Read the model definition and answer for the solid it produces. Units are mm, in the model's axes. A direction names the side the tool comes from. Coordinates: 2 decimals unless noted, no trailing zeros. Write each loop counter-clockwise with the first axis right and the second up, starting at its lowest first coordinate (ties: lowest second). Pieces come first, ordered by that corner, then holes.
(1) The part is cut by section C-C, the plane x = -3.5. Determine the outline of the cut face in (y, z), and give its area (3 significant figures).
(2) Straight lines are drawn through the part: line 1 along X through (y, z) = (-6, 5.5); line 2 along Z through (x, y) = (3, -7.25); line 3 along X through (y, z) = (-10, -0.25). For each, find the intervals that lie inside material, in ascending order.
(3) Given pin 1 (0.6 mm diameter, centred on x = -6, z = -5.5, fed in from -Y); pin 2 (0.5 mm diameter, centred on x = -6, z = 1.5, fed in from -Y); pin 3 (3 mm diameter, centred on x = -10.5, z = 2.5, fed in from -Y), each flat-ended and moving along its own axis, determine where each tip first touches the part or whether it passes through.
(4) Which of the six approach directions +Z, -Z, +X, -X, +Y, -Y give full straight-line access (tool end or side, diameter ignored) to faces 1 (the flat face through (-21, -7, 0)), 2 (the flat face through (-19, -6, -5.3)), 3 (the flat face through (0, 0, 0))?
(5) The part is cut by section B-B, the plane y = -4. Determine the outline of the cut face in (x, z), and give its area (3 significant figures).
(6) The part is cut by section A-A, the plane y = -6. State how many separate pieces and enclosed holes the cut face has, and give its area (3 significant figures).
(7) Determine the mould class of faces 4 (the flat face through (6.3, -4, 0)), 5 (the flat face through (3.16, -13, 7.15)) for opening direction Z: pulls with the +Z half, pulls with the -Z half, needs draft (parallel to the pull), parting line crosses it, or undercut.
(8) The part is cut by section D-D, the plane z = -1. Determine the outline of the cut face in (x, y).
```python
from build123d import *

# Parameters (mm, degrees)
SKETCH_1_W                             = 44
SKETCH_1_H                             = 16
EXTRUDE_1_DEPTH                        = 2
SKETCH_2_W                             = 44
SKETCH_2_H                             = 16
SKETCH_2_W_2                           = 40
SKETCH_2_H_2                           = 12
EXTRUDE_2_DEPTH                        = 10
SKETCH_3_W                             = 5.5
SKETCH_3_H                             = 4
CUT_EXTRUDE_1_DEPTH                    = 2
SKETCH_4_W                             = 1.7
SKETCH_4_H                             = 12
EXTRUDE_4_DEPTH                        = 4.6
SKETCH_9_W                             = 44
SKETCH_9_H                             = 16
SKETCH_9_W_2                           = 42
SKETCH_9_H_2                           = 14
EXTRUDE_5_DEPTH                        = 1
SKETCH_12_W                            = 1
SKETCH_12_H                            = 12
CUT_EXTRUDE_3_DEPTH                    = 5
SKETCH_13_W                            = 41.2
SKETCH_13_H                            = 13.2
SKETCH_13_W_2                          = 40
SKETCH_13_H_2                          = 12
REVB_ASSEMBLYCLEARANCE_41P2X13P2_DEPTH = 11
SKETCH_14_W                            = 11
SKETCH_14_H                            = 7
REVB_USB_TOPLOADING_USLOT_DEPTH        = 2.1
SKETCH_17_W                            = 10.6
SKETCH_17_H                            = 1.01
REVB_UNDERSIDESOLDERRELIEF_1MM_DEPTH   = 28


with BuildPart() as part:
    # 草图1 → 凸台-拉伸1 (new body)
    with BuildSketch(Plane(origin=(0, 0, 0), x_dir=(1, 0, 0), z_dir=(0, 1, 0))):
        Rectangle(SKETCH_1_W, SKETCH_1_H)
    extrude(amount=-EXTRUDE_1_DEPTH)

    # 草图2 → 凸台-拉伸2 (add)
    with BuildSketch(Plane.XZ.offset(2)):
        Rectangle(SKETCH_2_W, SKETCH_2_H)
        Rectangle(SKETCH_2_W_2, SKETCH_2_H_2, mode=Mode.SUBTRACT)
    extrude(amount=EXTRUDE_2_DEPTH)

    # 草图3 → 切除-拉伸1 (cut)
    with BuildSketch(Plane.ZY.offset(22)):
        with Locations((2.75, -9)):
            Rectangle(SKETCH_3_W, SKETCH_3_H)
        with Locations((-2.75, -9)):
            Rectangle(SKETCH_3_W, SKETCH_3_H)
    extrude(amount=-CUT_EXTRUDE_1_DEPTH, mode=Mode.SUBTRACT)

    # 草图4 → 凸台-拉伸4 (add)
    with BuildSketch(Plane.XZ.offset(2)):
        with Locations((7.15, 0)):
            Rectangle(SKETCH_4_W, SKETCH_4_H)
        with Locations((-19.15, 0)):
            Rectangle(SKETCH_4_W, SKETCH_4_H)
        with Locations((-6, 0)):
            Rectangle(SKETCH_4_W, SKETCH_4_H)
    extrude(amount=EXTRUDE_4_DEPTH)

    # 草图9 → 凸台-拉伸5 (add)
    with BuildSketch(Plane.XZ.offset(12)):
        Rectangle(SKETCH_9_W, SKETCH_9_H)
        Rectangle(SKETCH_9_W_2, SKETCH_9_H_2, mode=Mode.SUBTRACT)
    extrude(amount=EXTRUDE_5_DEPTH)

    # 草图12 → 切除-拉伸3 (cut)
    with BuildSketch(Plane.XZ.offset(12)):
        with Locations((20.5, 0)):
            Rectangle(SKETCH_12_W, SKETCH_12_H)
    extrude(amount=-CUT_EXTRUDE_3_DEPTH, mode=Mode.SUBTRACT)

    # 草图13 → RevB_AssemblyClearance_41p2x13p2 (cut)
    with BuildSketch(Plane.XZ.offset(13)):
        Rectangle(SKETCH_13_W, SKETCH_13_H)
        Rectangle(SKETCH_13_W_2, SKETCH_13_H_2, mode=Mode.SUBTRACT)
    extrude(amount=-REVB_ASSEMBLYCLEARANCE_41P2X13P2_DEPTH, mode=Mode.SUBTRACT)

    # 草图14 → RevB_USB_TopLoading_Uslot (cut)
    with BuildSketch(Plane.ZY.offset(22)):
        with Locations((0, -10.5)):
            Rectangle(SKETCH_14_W, SKETCH_14_H)
    extrude(amount=-REVB_USB_TOPLOADING_USLOT_DEPTH, mode=Mode.SUBTRACT)

    # 草图17 → RevB_UndersideSolderRelief_1mm (cut)
    with BuildSketch(Plane(origin=(8, 0, 0), x_dir=(0, 0, -1), z_dir=(1, 0, 0))):
        with Locations((0, -6.105)):
            Rectangle(SKETCH_17_W, SKETCH_17_H)
    extrude(amount=-REVB_UNDERSIDESOLDERRELIEF_1MM_DEPTH, mode=Mode.SUBTRACT)


solid = part.part
```
Computed:
1. outline: (-13, -8) - (0, -8) - (0, 8) - (-13, 8) - (-13, 7) - (-12, 7) - (-12, 6.6) - (-2, 6.6) - (-2, -6.6) - (-12, -6.6) - (-12, -7) - (-13, -7) - close
1. area: 62.0 mm2
2. line 1: x = -22 to -20.6, -20 to -18.3, -6.85 to -5.15, 6.3 to 8, 20.6 to 22
2. line 2: z = -8 to -6.6, 6.6 to 8
2. line 3: x = 21 to 22
3. pin 1: stops at y = -6.6
3. pin 2: stops at y = -5.6
3. pin 3: stops at y = -2
4. face 1: -X, -Y
4. face 2: -Y
4. face 3: +Z, -Z, +X, -X, +Y
5. outline: (-22, -8) - (22, -8) - (22, 8) - (-22, 8) - close; (-20, -6) - (-18.3, -6) - (-18.3, 6) - (-20, 6) - close; (-6.85, -6) - (-5.15, -6) - (-5.15, 6) - (-6.85, 6) - close; (6.3, -6) - (8, -6) - (8, 6) - (6.3, 6) - close; hole (-20.6, -6.6) - (20.6, -6.6) - (20.6, 6.6) - (-20.6, 6.6) - close
5. area: 221 mm2
6. separate pieces: 7
6. enclosed holes: 1
6. area: 167 mm2
7. face 4: undercut
7. face 5: needs draft
8. outline: (-22, -7) - (-20.6, -7) - (-20.6, -2) - (-20, -2) - (-20, -5.6) - (-18.3, -5.6) - (-18.3, -2) - (-6.85, -2) - (-6.85, -5.6) - (-5.15, -5.6) - (-5.15, -2) - (6.3, -2) - (6.3, -5.6) - (8, -5.6) - (8, -2) - (20.6, -2) - (20.6, -7) - (21, -7) - (21, -13) - (22, -13) - (22, 0) - (-22, 0) - close
